from build123d import *

# Parameters (mm, degrees)
BOSS_EXTRUDE1_DEPTH = 2.794
FILLET1_R           = 2.54
FILLET2_R           = 5.08
SKETCH2_W           = 6.35
SKETCH2_H           = 2.794
SKETCH2_W_2         = 2.794
SKETCH2_H_2         = 6.35
SKETCH2_H_3         = 1.5875
CUT_EXTRUDE1_DEPTH  = 73.220895192


with BuildPart() as part:
    # Sketch1 → Boss-Extrude1 (new body)
    with BuildSketch(Plane.XY):
        Polygon((-69.475359958, -4.3815), (18.662640042, -4.3815), (18.662640042, 19.525), (-0.387359958, 19.525), (-0.387359958, 8.3185), (-50.425359958, 8.3185), (-50.425359958, 19.525), (-69.475359958, 19.525), align=None)
    extrude(amount=BOSS_EXTRUDE1_DEPTH)

    # Fillet1
    fillet1_edges = [part.edges().sort_by_distance(p)[0] for p in [
        (18.662640042, -4.3815, 1.397),
        (-69.475359958, -4.3815, 1.397),
        (-69.475359958, 19.525, 1.397),
        (18.662640042, 19.525, 1.397),
    ]]
    fillet(fillet1_edges, radius=FILLET1_R)

    # Fillet2
    fillet2_edges = [part.edges().sort_by_distance(p)[0] for p in [
        (-50.425359958, 19.525, 1.397),
        (-50.425359958, 8.3185, 1.397),
        (-0.387359958, 8.3185, 1.397),
        (-0.387359958, 19.525, 1.397),
    ]]
    fillet(fillet2_edges, radius=FILLET2_R)

    # Sketch2 → Cut-Extrude1 (cut, through all)
    with BuildSketch(Plane.XY.offset(2.794)):
        with Locations((-47.250359958, -1.397)):
            Rectangle(SKETCH2_W, SKETCH2_H)
        with Locations((-3.562359958, -1.397)):
            Rectangle(SKETCH2_W, SKETCH2_H)
        with Locations((15.678140042, 9.525)):
            Rectangle(SKETCH2_W_2, SKETCH2_H_2)
        with Locations((-66.490859958, 9.525)):
            Rectangle(SKETCH2_W_2, SKETCH2_H_2)
        with Locations((5.962640042, 2.38125)):
            Rectangle(SKETCH2_W, SKETCH2_H_3)
        with Locations((-56.775359958, 2.38125)):
            Rectangle(SKETCH2_W, SKETCH2_H_3)
    extrude(amount=-CUT_EXTRUDE1_DEPTH, mode=Mode.SUBTRACT)


solid = part.part
Geometry: final body of the model. Coordinates: model frame, mm. A direction names the side the tool comes from. Round coordinates to 2 decimals unless told otherwise and drop trailing zeros. Loops run counter-clockwise (first coordinate to the right, second up) from the corner with the lowest first, then second, coordinate; pieces in that order, holes last.
Q1. Section B-B on y = 10.75. Return loops of the section in (x, z), plus the area to 3 significant figures.
Q2. Pull-direction query (Y, two-part tool) for faces 4 (the flat face through (-69.475, 8, 1)), 5 (the cylindrical face through (-1.836, 9.846, 1.417)), 6 (the flat face through (-50.425, -1, 1)); classes: released by +Y, released by -Y, zero draft, split by the parting line, or undercut.
Q3. Section D-D on x = -21. Return loops of the section in (y, z), plus the area to 3 significant figures.
Q4. Access query for faces 1 (the flat face through (-25, 8.318, 1)), 2 (the flat face through (-47, 0, 1)), 3 (the flat face through (-26, 5, 0)). Directions: +Z, -Z, +X, -X, +Y, -Y. A direction counts if a zero-diameter tool reaches every point of the face in a straight line with its end or side. Return the directions, or none.
Q5. Pin query (flat end, axial travel): P1, Ø1.4, axis at x = -2.5, z = 2, coming from the +Y side; P2, Ø1, axis at x = -31, z = 2.5, coming from the +Y side. Return the tip coordinate at first contact, or that it passes through.
Q6. Section C-C on y = 15.5. Return loops of the section in (x, z).
Q7. Section A-A on x = -4.5. Return loops of the section in (y, z).
Q8. Material intervals for L1, parallel to X at y = 6.5, z = 0.3; L2, parallel to Y at x = -58, z = 1.9 (1 decimal); L3, parallel to Y at x = -25, z = 2.4, sorted ascending.
Evaluation:
1. outline: (-69.48, 0) - (-67.89, 0) - (-67.89, 2.79) - (-69.48, 2.79) - close; (-65.09, 0) - (-49.68, 0) - (-49.68, 2.79) - (-65.09, 2.79) - close; (-1.13, 0) - (14.28, 0) - (14.28, 2.79) - (-1.13, 2.79) - close; (17.08, 0) - (18.66, 0) - (18.66, 2.79) - (17.08, 2.79) - close
1. area: 95.0 mm2
2. face 4: zero draft
2. face 5: released by +Y
2. face 6: undercut
3. outline: (-4.38, 0) - (8.32, 0) - (8.32, 2.79) - (-4.38, 2.79) - close
3. area: 35.5 mm2
4. face 1: +Z, -Z, +Y
4. face 2: +Z, -Z
4. face 3: -Z, +X, -X, +Y, -Y
5. P1: stops at y = 9.88
5. P2: stops at y = 8.32
6. outline: (-69.48, 0) - (-50.54, 0) - (-50.54, 2.79) - (-69.48, 2.79) - close; (-0.28, 0) - (18.66, 0) - (18.66, 2.79) - (-0.28, 2.79) - close
7. outline: (-4.38, 0) - (-2.79, 0) - (-2.79, 2.79) - (-4.38, 2.79) - close; (0, 0) - (8.41, 0) - (8.41, 2.79) - (0, 2.79) - close
8. L1: x = -69.48 to -67.89, -65.09 to 14.28, 17.08 to 18.66
8. L2: y = -4.4 to 1.6, 3.2 to 19.5
8. L3: y = -4.38 to 8.32
